The model under review builds one solid part; all positions refer to its coordinate system, in mm. Coordinates: 2 decimals unless noted, no trailing zeros. Order: outer loops, then holes, each group sorted by start corner. A loop starts at its lowest first (then second) coordinate and runs counter-clockwise, first axis right, second up. Notation, with made-up numbers: (15, 56.25) -> (20, 56.25) arc R22 cw to (20, 84.25) -> close; hole circle Ø2 at (-5, 61). An arc over 180 degrees is marked (long way). Use one line per item in the form item = value.
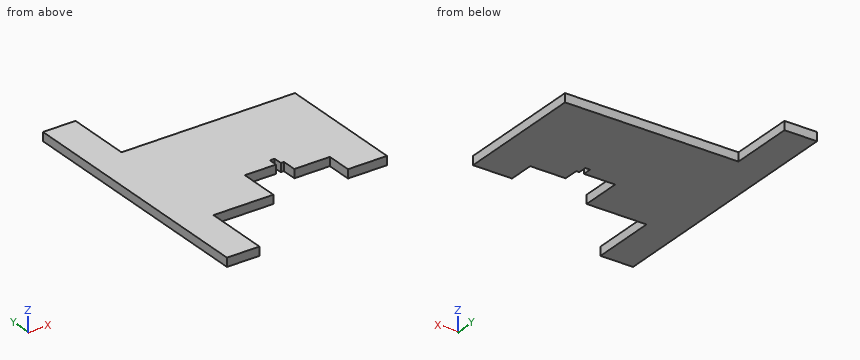
from build123d import *

# Parameters (mm, degrees)
BOSS_EXTRUDE1_DEPTH     = 5.08
CUT_EXTRUDE1_DEPTH      = 154.012602095
CUT_EXTRUDE1_DEPTH_BACK = 154.012602095


with BuildPart() as part:
    # Sketch1 → Boss-Extrude1 (new body)
    with BuildSketch(Plane.XY):
        Polygon((0, 0), (101.6, 0), (101.6, -76.2), (0, -76.2), (0, -114.3), (-19.05, -114.3), (-19.05, 38.1), (0, 38.1), align=None)
    extrude(amount=BOSS_EXTRUDE1_DEPTH)

    # Sketch2 → Cut-Extrude1 (cut, two sides: drawn at the far end of the back side and taken through both)
    with BuildSketch(Plane.XY.offset(5.08).offset(-CUT_EXTRUDE1_DEPTH_BACK)):
        Polygon((35.052, -76.2), (35.052, -52.578), (53.34, -52.578), (53.34, -47.498), (56.134, -47.498), (56.134, -52.578), (57.912, -52.578), (57.912, -61.214), (78.74, -61.214), (78.74, -76.2), align=None)
    extrude(amount=CUT_EXTRUDE1_DEPTH + CUT_EXTRUDE1_DEPTH_BACK, mode=Mode.SUBTRACT)


solid = part.part
Item 1: To check wall thickness, follow L1, parallel to X at y = -57, z = 2.5; L2, parallel to X at y = -61.5, z = 0.95; L3, parallel to X at y = 31, z = 4. State the ranges of each line that lie inside material, in increasing order. Write a range as from..to.
Results found:
L1 = -19.05..35.05, 57.91..101.6
L2 = -19.05..35.05, 78.74..101.6
L3 = -19.05..0
Item 2: We need section B-B (z = 4.1). Write out the cut boundary in (x, y).
Results found:
outline = (-19.05, -114.3) -> (0, -114.3) -> (0, -76.2) -> (35.05, -76.2) -> (35.05, -52.58) -> (53.34, -52.58) -> (53.34, -47.5) -> (56.13, -47.5) -> (56.13, -52.58) -> (57.91, -52.58) -> (57.91, -61.21) -> (78.74, -61.21) -> (78.74, -76.2) -> (101.6, -76.2) -> (101.6, 0) -> (0, 0) -> (0, 38.1) -> (-19.05, 38.1) -> close
Item 3: We need section D-D (y = -96). Write out the cut boundary in (x, z), plus the area to 3 significant figures.
Results found:
outline = (-19.05, 0) -> (0, 0) -> (0, 5.08) -> (-19.05, 5.08) -> close
area = 96.8 mm²
Item 4: We need section C-C (x = 30.5). Write out the cut boundary in (y, z), plus the area to 3 significant figures.
Results found:
outline = (-76.2, 0) -> (0, 0) -> (0, 5.08) -> (-76.2, 5.08) -> close
area = 387 mm²
Item 5: Clearance check with flat-ended pins moving along their axes: pin 1 (1.4 mm diameter, centred on x = 54, z = 3, fed in from -Y); pin 2 (1.5 mm diameter, centred on x = 66.5, z = 2, fed in from -Y); pin 3 (2.5 mm diameter, centred on x = 72, z = 2, fed in from +Y). State where each tip first meets the part, or that it passes through.
Results found:
pin_1 = -52.58
pin_2 = -61.21
pin_3 = 0
Item 6: We need section A-A (y = -65). Write out the cut boundary in (x, z), plus the area to 3 significant figures.
Results found:
outline = (-19.05, 0) -> (35.05, 0) -> (35.05, 5.08) -> (-19.05, 5.08) -> close; (78.74, 0) -> (101.6, 0) -> (101.6, 5.08) -> (78.74, 5.08) -> close
area = 391 mm²
